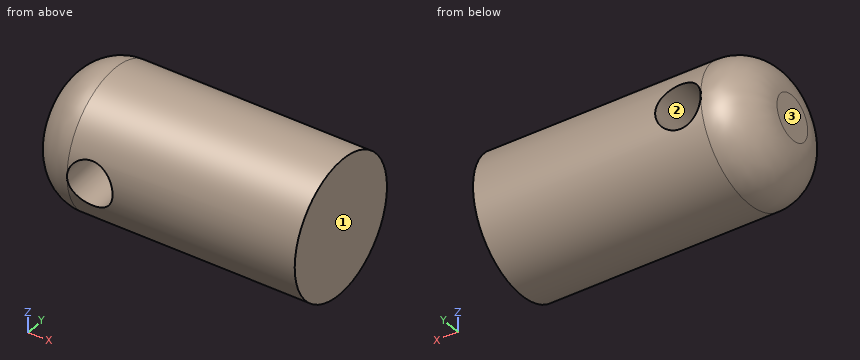
```python
from build123d import *

# Parameters (mm, degrees)
F0_R     = 19.05
F1_DEPTH = 25.4
F2_DEPTH = 25.4
F4_R     = 12.7
F3_R     = 6.35
F5_DEPTH = 19.05


with BuildPart() as f1:
    # F0 (on Right) → F1 (new body, symmetric)
    with BuildSketch(Plane.YZ):
        Circle(F0_R)
    extrude(amount=F1_DEPTH, both=True)

    # F2 (add): a face of the model
    f2_faces = [f1.faces().sort_by_distance(p)[0] for p in [
        (-25.4, 0, 0),
    ]]
    extrude(f2_faces, amount=F2_DEPTH)

    # F4
    f4_edges = [f1.edges().sort_by_distance(p)[0] for p in [
        (-50.8, -19.05, 0),
    ]]
    fillet(f4_edges, radius=F4_R)

    # F3 (on Front) → F5 (cut, symmetric)
    with BuildSketch(Plane.XZ):
        with Locations((-31.75, 0)):
            Circle(F3_R)
    extrude(amount=F5_DEPTH, both=True, mode=Mode.SUBTRACT)


solid = f1.part
```
CAD build for the part. Positions are in the model's coordinates, mm. Face numbers are marked on the shaded views. Coordinates: 2 decimals unless noted, no trailing zeros. Loops run counter-clockwise (first coordinate to the right, second up) from the corner with the lowest first, then second, coordinate; pieces in that order, holes last. Notation, with made-up numbers: (54, -37) - (101, -37) arc R18 cw to (101, -11) - close; hole circle Ø1 at (37.25, 24.5). An arc over 180 degrees is marked (long way). Return JSON: item names as keys, results as strings.
1. Band-saw the part on A-A (x = -31.75). Give the cut face in (y, z), and give its area (3 significant figures).
Result:
{"outline": "(-17.96, -6.35) arc R19.05 ccw to (17.96, -6.35) - close; (-17.96, 6.35) - (17.96, 6.35) arc R19.05 ccw to start", "area": "665 mm2"}
2. Mould opens along X. For the marked faces 1, 2 and 3 say: released by +X, released by -X, zero draft, split by the parting line, or undercut.
Result:
{"face 1": "released by +X", "face 2": "undercut", "face 3": "released by -X"}
3. Probe L1, parallel to X at y = -0.5, z = 0; L2, parallel to Z at x = -29.5, y = 1.5; L3, parallel to X at y = 13.5, z = -2.5. List the from-to ranges inside material, lowest first. Write a range as from..to.
Result:
{"L1": "x = -50.8..-38.1, -25.4..25.4", "L2": "z = -18.99..-5.94, 5.94..18.99", "L3": "x = -48.44..-37.59, -25.91..25.4"}
4. Drop flat-ended pins along their axis: pin 1 (1 mm diameter, centred on x = 4, y = 8, fed in from +Z); pin 2 (1 mm diameter, centred on x = 16.5, z = -13, fed in from -Y); pin 3 (1 mm diameter, centred on x = -18, z = 2, fed in from -Y). Give the stop position or say it passes through.
Result:
{"pin 1": "stops at z = 17.51", "pin 2": "stops at y = -14.38", "pin 3": "stops at y = -18.99"}
5. Band-saw the part on B-B (x = -1). Give the cut face in (y, z).
Result:
{"outline": "circle Ø38.1 at (0, 0)"}
